Part model, mm, in its own coordinate system. Face numbers are marked on the shaded views. A direction names the side the tool comes from. Round coordinates to 2 decimals unless told otherwise and drop trailing zeros. Write each loop counter-clockwise with the first axis right and the second up, starting at its lowest first coordinate (ties: lowest second). Pieces come first, ordered by that corner, then holes. Notation, with made-up numbers: M -20,-4 L 33,-4 A30 ccw 33,24 Z; hole C 87,21 d7. An arc over 180 degrees is marked long. Use a Markdown table: item, result. Add a question column.
1) Drop flat-ended pins along their axis: P1, Ø3.5, axis at x = -8, z = 0, coming from the +Y side; P2, Ø3, axis at x = -11.5, z = 3.5, coming from the -Y side. Give the stop position or say it passes through.
2) Slice it at C-C on z = 6. Write the cut outline in (x, y).
3) Which spindle directions (+Z, -Z, +X, -X, +Y, -Y) get a long thin tool onto all of the face, cutting with end or side? Do the marked faces 1, 2 and 3. Say none if no direction does.
4) Slice it at A-A on y = 7. Give the number of separate pieces and of enclosed holes in the cut face, plus the area to 3 significant figures.
5) Two-plate mould, pull along Z, no slides. Class the marked faces 4, 5 and 6: released by +Z, released by -Z, zero draft, split by the parting line, or undercut.
6) Wall check: probe 1 along X at (y, z) = (9.45, -4); probe 2 along X at (y, z) = (6, 3.5); probe 3 along X at (y, z) = (6.75, -6). Give the ranges that are in metal, low to high.
7) Slice it at B-B on x = 0. Write the cut outline in (y, z).
8) Slice it at D-D on x = 12. Write the cut outline in (y, z), plus the area to 3 significant figures.
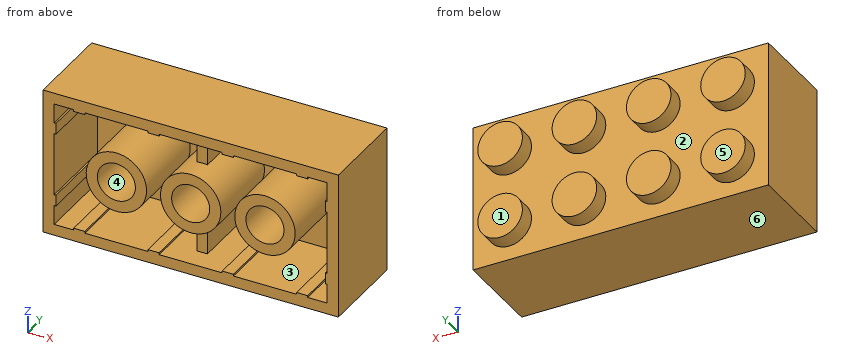
```python
from build123d import *

# Parameters (mm, degrees)
SKETCH1_W           = 31.8
SKETCH1_H           = 15.8
BOSS_EXTRUDE1_DEPTH = 9.6
SKETCH2_R           = 2.4
BOSS_EXTRUDE2_DEPTH = 1.8
CUT_EXTRUDE8_DEPTH  = 8.6
SKETCH5_R           = 1.3
CUT_EXTRUDE9_DEPTH  = 1.7
SKETCH6_R           = 3.25
SKETCH6_R_2         = 2.05
BOSS_EXTRUDE3_DEPTH = 8.6
BOSS_EXTRUDE4_DEPTH = 6.3


with BuildPart() as part:
    # Sketch1 → Boss-Extrude1 (new body)
    with BuildSketch(Plane(origin=(0, 0, 0), x_dir=(1, 0, 0), z_dir=(0, 1, 0))):
        Rectangle(SKETCH1_W, SKETCH1_H)
    extrude(amount=BOSS_EXTRUDE1_DEPTH)

    # Sketch2 → Boss-Extrude2 (add)
    with BuildSketch(Plane(origin=(0, 9.6, 0), x_dir=(1, 0, 0), z_dir=(0, 1, 0))):
        with Locations(Location((-4, 4, 0), (0, 0, 270))):
            Circle(SKETCH2_R)
        with Locations(Location((-12, 4, 0), (0, 0, 270))):
            Circle(SKETCH2_R)
        with Locations(Location((4, 4, 0), (0, 0, 270))):
            Circle(SKETCH2_R)
        with Locations(Location((12, 4, 0), (0, 0, 270))):
            Circle(SKETCH2_R)
        with Locations(Location((12, -4, 0), (0, 0, 90))):
            Circle(SKETCH2_R)
        with Locations(Location((4, -4, 0), (0, 0, 90))):
            Circle(SKETCH2_R)
        with Locations(Location((-4, -4, 0), (0, 0, 90))):
            Circle(SKETCH2_R)
        with Locations(Location((-12, -4, 0), (0, 0, 90))):
            Circle(SKETCH2_R)
    extrude(amount=BOSS_EXTRUDE2_DEPTH)

    # Sketch4 → Cut-Extrude8 (cut)
    with BuildSketch(Plane(origin=(0, 0, 0), x_dir=(-1, 0, 0), z_dir=(0, -1, 0))):
        Polygon((14.7, 3.398716226), (14.7, -3.398716226), (14.5, -3.398716226), (14.5, -4.601283774), (14.7, -4.601283774), (14.7, -6.7), (12.6, -6.7), (12.6, -6.5), (11.4, -6.5), (11.4, -6.7), (4.601283774, -6.7), (4.601283774, -6.5), (3.398716226, -6.5), (3.398716226, -6.7), (-3.398716226, -6.7), (-3.398716226, -6.5), (-4.601283774, -6.5), (-4.601283774, -6.7), (-11.4, -6.7), (-11.4, -6.5), (-12.6, -6.5), (-12.6, -6.7), (-14.7, -6.7), (-14.7, -4.601283774), (-14.5, -4.601283774), (-14.5, -3.398716226), (-14.7, -3.398716226), (-14.7, 3.398716226), (-14.5, 3.398716226), (-14.5, 4.601283774), (-14.7, 4.601283774), (-14.7, 6.7), (-12.6, 6.7), (-12.6, 6.5), (-11.4, 6.5), (-11.4, 6.7), (-4.601283774, 6.7), (-4.601283774, 6.5), (-3.398716226, 6.5), (-3.398716226, 6.7), (3.398716226, 6.7), (3.398716226, 6.5), (4.601283774, 6.5), (4.601283774, 6.7), (11.4, 6.7), (11.4, 6.5), (12.6, 6.5), (12.6, 6.7), (14.7, 6.7), (14.7, 4.601283774), (14.5, 4.601283774), (14.5, 3.398716226), align=None)
    extrude(amount=-CUT_EXTRUDE8_DEPTH, mode=Mode.SUBTRACT)

    # Sketch5 → Cut-Extrude9 (cut)
    with BuildSketch(Plane(origin=(0, 8.6, 0), x_dir=(-1, 0, 0), z_dir=(0, -1, 0))):
        with Locations(Location((12, -4, 0), (0, 0, 90))):
            Circle(SKETCH5_R)
        with Locations(Location((4, -4, 0), (0, 0, 90))):
            Circle(SKETCH5_R)
        with Locations(Location((-4, -4, 0), (0, 0, 90))):
            Circle(SKETCH5_R)
        with Locations(Location((-12, -4, 0), (0, 0, 90))):
            Circle(SKETCH5_R)
        with Locations(Location((4, 4, 0), (0, 0, 90))):
            Circle(SKETCH5_R)
        with Locations(Location((-4, 4, 0), (0, 0, 90))):
            Circle(SKETCH5_R)
        with Locations(Location((-12, 4, 0), (0, 0, 90))):
            Circle(SKETCH5_R)
        with Locations(Location((12, 4, 0), (0, 0, 90))):
            Circle(SKETCH5_R)
    extrude(amount=-CUT_EXTRUDE9_DEPTH, mode=Mode.SUBTRACT)

    # Sketch6 → Boss-Extrude3 (add)
    # profile 1 of 3: a face of its own
    with BuildSketch(Plane(origin=(0, 8.6, 0), x_dir=(-1, 0, 0), z_dir=(0, -1, 0))):
        with Locations(Location((0, 0, 0), (0, 0, 270))):
            Circle(SKETCH6_R)
        with Locations(Location((0, 0, 0), (0, 0, 270))):
            Circle(SKETCH6_R_2, mode=Mode.SUBTRACT)
    # profile 2 of 3: a face of its own
    with BuildSketch(Plane(origin=(0, 8.6, 0), x_dir=(-1, 0, 0), z_dir=(0, -1, 0))):
        with Locations(Location((8, 0, 0), (0, 0, 270))):
            Circle(SKETCH6_R)
        with Locations(Location((8, 0, 0), (0, 0, 270))):
            Circle(SKETCH6_R_2, mode=Mode.SUBTRACT)
    # profile 3 of 3: a face of its own
    with BuildSketch(Plane(origin=(0, 8.6, 0), x_dir=(-1, 0, 0), z_dir=(0, -1, 0))):
        with Locations(Location((-8, 0, 0), (0, 0, 270))):
            Circle(SKETCH6_R)
        with Locations(Location((-8, 0, 0), (0, 0, 270))):
            Circle(SKETCH6_R_2, mode=Mode.SUBTRACT)
    extrude(amount=BOSS_EXTRUDE3_DEPTH)

    # Sketch7 → Boss-Extrude4 (add)
    with BuildSketch(Plane(origin=(0, 8.6, 0), x_dir=(-1, 0, 0), z_dir=(0, -1, 0))):
        with BuildLine():
            Line((0.55, -3.203123476), (0.55, -6.7))
            Line((0.55, -6.7), (-0.55, -6.7))
            Line((-0.55, -6.7), (-0.55, -3.203123476))
            ThreePointArc((-0.55, -3.203123476), (0, -3.25), (0.55, -3.203123476))
        make_face()
        with BuildLine():
            Line((-0.55, 6.7), (-0.55, 3.203123476))
            ThreePointArc((-0.55, 3.203123476), (0, 3.25), (0.55, 3.203123476))
            Line((0.55, 3.203123476), (0.55, 6.7))
            Line((0.55, 6.7), (-0.55, 6.7))
        make_face()
    extrude(amount=BOSS_EXTRUDE4_DEPTH)


solid = part.part
```
Entries:
| question | item | result |
|---|---|---|
| 1 | P1 | stops at y = 9.6 |
| 1 | P2 | stops at y = 8.6 |
| 2 | outline | M -15.9,0 L -14.7,0 L -14.7,8.6 L -0.55,8.6 L -0.55,2.3 L 0.55,2.3 L 0.55,8.6 L 14.7,8.6 L 14.7,0 L 15.9,0 L 15.9,9.6 L 13.33,9.6 L 13.33,11.4 L 10.67,11.4 L 10.67,9.6 L 5.33,9.6 L 5.33,11.4 L 2.67,11.4 L 2.67,9.6 L -2.67,9.6 L -2.67,11.4 L -5.33,11.4 L -5.33,9.6 L -10.67,9.6 L -10.67,11.4 L -13.33,11.4 L -13.33,9.6 L -15.9,9.6 Z |
| 3 | face 1 | +Z, -Z, +X, -X, +Y |
| 3 | face 2 | +Y |
| 3 | face 3 | -Y |
| 4 | separate pieces | 3 |
| 4 | enclosed holes | 5 |
| 4 | area | 179 mm^2 |
| 5 | face 4 | undercut |
| 5 | face 5 | zero draft |
| 5 | face 6 | released by -Z |
| 6 | probe 1 | x = -15.9 to -13.3, -10.7 to -5.3, -2.7 to 2.7, 5.3 to 10.7, 13.3 to 15.9 |
| 6 | probe 2 | x = -15.9 to -14.5, -0.55 to 0.55, 14.5 to 15.9 |
| 6 | probe 3 | x = -15.9 to -14.7, -0.55 to 0.55, 14.7 to 15.9 |
| 7 | outline | M 0,-7.9 L 9.6,-7.9 L 9.6,7.9 L 0,7.9 L 0,6.7 L 2.3,6.7 L 2.3,3.25 L 0,3.25 L 0,2.05 L 8.6,2.05 L 8.6,-2.05 L 0,-2.05 L 0,-3.25 L 2.3,-3.25 L 2.3,-6.7 L 0,-6.7 Z |
| 8 | outline | M 0,-7.9 L 9.6,-7.9 L 9.6,-6.4 L 11.4,-6.4 L 11.4,-1.6 L 9.6,-1.6 L 9.6,1.6 L 11.4,1.6 L 11.4,6.4 L 9.6,6.4 L 9.6,7.9 L 0,7.9 L 0,6.5 L 8.6,6.5 L 8.6,5.3 L 10.3,5.3 L 10.3,2.7 L 8.6,2.7 L 8.6,-2.7 L 10.3,-2.7 L 10.3,-5.3 L 8.6,-5.3 L 8.6,-6.5 L 0,-6.5 Z |
| 8 | area | 48.3 mm^2 |
